```python
from build123d import *

# Parameters (mm, degrees)
F0_W     = 10
F0_H     = 18.7
F1_DEPTH = 2
F2_W     = 10
F2_H     = 0.5
F3_DEPTH = 3.5
F4_R     = 3
F5_DEPTH = 25


with BuildPart() as f1:
    # F0 (on Front) → F1 (new body)
    with BuildSketch(Plane.XZ):
        Rectangle(F0_W, F0_H)
    extrude(amount=F1_DEPTH)

    # F2 (on face) → F3 (join)
    with BuildSketch(Plane.XZ.offset(2)):
        with Locations((0, 9.1)):
            Rectangle(F2_W, F2_H)
        with Locations((0, -9.1)):
            Rectangle(F2_W, F2_H)
    extrude(amount=F3_DEPTH)

    # F4 (on face) → F5 (cut)
    with BuildSketch(Plane(origin=(0, 0, 0), x_dir=(-1, 0, 0), z_dir=(0, 1, 0))):
        Circle(F4_R)
    extrude(amount=-F5_DEPTH, mode=Mode.SUBTRACT)


solid = f1.part
```
The listing builds one solid part. Answer for the finished solid, in the listing's coordinates (mm). A direction names the side the tool comes from. Coordinates: 2 decimals unless noted, no trailing zeros. Loops run counter-clockwise (first coordinate to the right, second up) from the corner with the lowest first, then second, coordinate; pieces in that order, holes last. Notation, with made-up numbers: (-10, 81.5) -> (0, 81.5) arc R17 cw to (0, 87.5) -> close; hole circle Ø1 at (44.5, 35). An arc over 180 degrees is marked (long way). Use one line per item in the form item = value. Start each with the question number.
Item 1: A tool of negligible diameter and unlimited length cuts with its end or side. For faces 5 (the face through (5, -1.5, 0)), 6 (the face through (3.3, -2, 0.1)), from which of +Z, -Z, +X, -X, +Y, -Y can it reach the whole face along a straight path? Write none if from no direction.
Item 2: The part is cut by section C-C on z = 0. Determine the outline of the cut face in (x, y), then the cut area to 3 significant figures.
Item 3: The part is cut by section D-D on y = -1.2. Determine the outline of the cut face in (x, z).
Item 4: The mould has two halves that part along Z. Classify faces 1 (the face through (0, -3, 9.35)), 2 (the face through (0, -4, -8.85)), 3 (the face through (3, -1, 0)), 4 (the face through (-5, -1.5, 0)): released by +Z, released by -Z, zero draft, split by the parting line, or undercut.
Item 5: The part is cut by section A-A on y = -2.8. Determine the outline of the cut face in (x, z), then the cut area to 3 significant figures.
Item 6: Consider L1, parallel to Z at x = 0, y = -1.5; L2, parallel to Z at x = -1, y = -2.7; L3, parallel to Y at x = 2.75, z = -6.75. Determine where each line is inside the solid, lowest interval first. Write a range as [from, to].
Item 7: The part is cut by section B-B on x = 0. Determine the outline of the cut face in (y, z).
Answer key:
q1.face_5 = +Z, -Z, +X, +Y, -Y
q1.face_6 = +X, -X, -Y
q2.outline = (-5, -2) -> (-3, -2) -> (-3, 0) -> (-5, 0) -> close; (3, -2) -> (5, -2) -> (5, 0) -> (3, 0) -> close
q2.area = 8.00 mm2
q3.outline = (-5, -9.35) -> (5, -9.35) -> (5, 9.35) -> (-5, 9.35) -> close; hole circle Ø6 at (0, 0)
q4.face_1 = released by +Z
q4.face_2 = undercut
q4.face_3 = undercut
q4.face_4 = zero draft
q5.outline = (-5, -9.35) -> (5, -9.35) -> (5, -8.85) -> (-5, -8.85) -> close; (-5, 8.85) -> (5, 8.85) -> (5, 9.35) -> (-5, 9.35) -> close
q5.area = 10.0 mm2
q6.L1 = [-9.35, -3], [3, 9.35]
q6.L2 = [-9.35, -8.85], [8.85, 9.35]
q6.L3 = [-2, 0]
q7.outline = (-5.5, -9.35) -> (0, -9.35) -> (0, -3) -> (-2, -3) -> (-2, -8.85) -> (-5.5, -8.85) -> close; (-5.5, 8.85) -> (-2, 8.85) -> (-2, 3) -> (0, 3) -> (0, 9.35) -> (-5.5, 9.35) -> close
